Autodesk Inventor part; units mm, degrees
ref_plane "YZ Plane" through (0, 0, 0) normal (1, 0, 0) x (0, 1, 0)
ref_plane "XZ Plane" through (0, 0, 0) normal (0, 1, 0) x (-1, 0, 0)
ref_plane "XY Plane" through (0, 0, 0) normal (0, 0, 1) x (1, 0, 0)
sketch "Sketch1" plane through (0, 0, 0) normal (0, 1, 0) x (-1, 0, 0)
  line L0 (0, 0) -> (-25, 0)
  line L1 (-25, 0) -> (-25, 25)
  line L2 (-25, 25) -> (0, 25)
  line L3 (0, 25) -> (0, 0)
  circle A0 centre (-4.5, 4.5) radius 3
  circle A1 centre (-4.5, 20.5) radius 3
  circle A2 centre (-20.5, 20.5) radius 3
  circle A3 centre (-20.5, 4.5) radius 3
  dimension "d0" = 25
  dimension "d1" = 25
  dimension "d8" = 6
  dimension "d9" = 6
  dimension "d10" = 6
  dimension "d11" = 6
extrude "Extrusion1" add sketch "Sketch1" along normal blind 1 contours L0 L1 L2 L3 | A0 | A1 | A2 | A3
sketch "Sketch2" plane through (0, 1, 0) normal (0, 1, 0) x (1, 0, 0)
  line L0 (10, -12.5) -> (10, -15)
  line L1 (10, -15) -> (12.5, -15)
  line L2 (10, -12.5) -> (10, -10)
  line L3 (10, -10) -> (12.5, -10)
  line L4 (15, -12.5) -> (15, -15)
  line L5 (15, -15) -> (12.5, -15)
  line L6 (15, -12.5) -> (15, -10)
  line L7 (15, -10) -> (12.5, -10)
  point P0 (0, 0)
  dimension "d18" = 2.5
  dimension "d19" = 2.5
  dimension "d20" = 2.5
  dimension "d21" = 2.5
  dimension "d22" = 2.5
  dimension "d23" = 2.5
extrude "Extrusion2" add sketch "Sketch2" along normal blind 0.5
sketch "Sketch6" plane through (0, 1, 0) normal (0, 1, 0) x (1, 0, 0)
  circle A0 centre (4.5, -4.5) radius 4
  circle A1 centre (20.5, -4.5) radius 4
  circle A2 centre (4.5, -20.5) radius 4
  circle A3 centre (20.5, -20.5) radius 4
  point P0 (0, 0)
  dimension "d43" = 8
  dimension "d44" = 8
  dimension "d45" = 8
  dimension "d46" = 8
extrude "Extrusion4" add sketch "Sketch6" along normal blind 0.25
sketch "Sketch7" plane through (4.5, 1.25, 20.5) normal (0, 1, 0) x (1, 0, 0)
  circle A0 centre (0, 0) radius 3
  point P0 (-4.5, 20.5)
  dimension "d49" = 6
hole "Hole2" at (4.5, 1.25, 20.5) direction (0, -1, 0) diameter 6 depth 1.25
sketch "Sketch8" plane through (4.5, 1.25, 4.5) normal (0, 1, 0) x (1, 0, 0)
  circle A0 centre (0, 0) radius 3
  point P0 (-4.5, 4.5)
  dimension "d57" = 6
hole "Hole3" at (4.5, 1.25, 4.5) direction (0, -1, 0) diameter 6 depth 1.25
sketch "Sketch9" plane through (20.5, 1.25, 20.5) normal (0, 1, 0) x (1, 0, 0)
  circle A0 centre (0, 0) radius 3
  point P0 (-20.5, 20.5)
  dimension "d65" = 6
hole "Hole4" at (20.5, 1.25, 20.5) direction (0, -1, 0) diameter 6 depth 1.25
sketch "Sketch10" plane through (20.5, 1.25, 4.5) normal (0, 1, 0) x (1, 0, 0)
  circle A0 centre (0, 0) radius 3
  point P0 (-20.5, 4.5)
  dimension "d73" = 6
hole "Hole5" at (20.5, 1.25, 4.5) direction (0, -1, 0) diameter 6 depth 1.25
properties part number "SiPM"
Can you work these out from the model? Positions are in its coordinate system, mm. A direction names the side the tool comes from. Coordinates: 2 decimals unless noted, no trailing zeros. Loops run counter-clockwise (first coordinate to the right, second up) from the corner with the lowest first, then second, coordinate; pieces in that order, holes last. Notation, with made-up numbers: (31.25, 1.5) -> (62.25, 1.5) arc R5 ccw to (62.25, 9.5) -> close; hole circle Ø2 at (-10, -21). An arc over 180 degrees is marked (long way). Put each result on its own line as item: value. Start each with the question number.
Q1. I'm going to push flat-ended pins straight in: P1, Ø1, axis at x = 10, z = 5.5, coming from the -Y side; P2, Ø4, axis at x = 6, z = 19.5, coming from the +Y side; P3, Ø2.5, axis at x = 19.5, z = 20.5, coming from the +Y side (1 decimal); P4, Ø1, axis at x = 4, z = 9.5, coming from the +Y side. Where does each tip first touch, or does it pass through?
Q2. I want a section at A-A (z = 4.5). Write out the boundary of the cut face in (x, y), plus the area to 3 significant figures.
Q3. If I drill on line 1 (Z direction, x = 4.5, y = 0.9); line 2 (X direction, y = 0.45, z = 2), over which ranges is the centre line in solid material (lowest first)? Write a range as [from, to].
Q4. I want a section at D-D (z = 12). Write out the boundary of the cut face in (x, y), plus the area to 3 significant figures.
Q5. I want a section at C-C (y = 0.35). Write out the boundary of the cut face in (x, z), plus the area to 3 significant figures.
Q6. I want a section at B-B (x = 4.5). Write out the boundary of the cut face in (y, z).
Q7. For faces 1 (the face through (15.5, 1, 12.7)), 2 (the face through (25, 0.5, 12.3)), which set-ups out of +Z, -Z, +X, -X, +Y, -Y let a thin tool reach every point of the face, with its end or its side?
Q8. Thinking about a two-plate mould opening in X: for faces 3 (the face through (12.3, 0.5, 0)), 4 (the face through (0, 0.5, 12.7)), 5 (the face through (22.3, 0.6, 18.1)), which applies, pulls with the +X half, pulls with the -X half, needs draft (parallel to the pull), parting line crosses it, or undercut?
Taken from the geometry:
1. P1: stops at y = 0
1. P2: stops at y = 1.25
1. P3: passes through
1. P4: stops at y = 1
2. outline: (0, 0) -> (1.5, 0) -> (1.5, 1.25) -> (0.5, 1.25) -> (0.5, 1) -> (0, 1) -> close; (7.5, 0) -> (17.5, 0) -> (17.5, 1.25) -> (16.5, 1.25) -> (16.5, 1) -> (8.5, 1) -> (8.5, 1.25) -> (7.5, 1.25) -> close; (23.5, 0) -> (25, 0) -> (25, 1) -> (24.5, 1) -> (24.5, 1.25) -> (23.5, 1.25) -> close
2. area: 14.0 mm2
3. line 1: z = [0, 1.5], [7.5, 17.5], [23.5, 25]
3. line 2: x = [0, 2.84], [6.16, 18.84], [22.16, 25]
4. outline: (0, 0) -> (25, 0) -> (25, 1) -> (15, 1) -> (15, 1.5) -> (10, 1.5) -> (10, 1) -> (0, 1) -> close
4. area: 27.5 mm2
5. outline: (0, 0) -> (25, 0) -> (25, 25) -> (0, 25) -> close; hole circle Ø6 at (4.5, 4.5); hole circle Ø6 at (4.5, 20.5); hole circle Ø6 at (20.5, 4.5); hole circle Ø6 at (20.5, 20.5)
5. area: 512 mm2
6. outline: (0, 0) -> (1, 0) -> (1, 0.5) -> (1.25, 0.5) -> (1.25, 1.5) -> (0, 1.5) -> close; (0, 7.5) -> (1.25, 7.5) -> (1.25, 8.5) -> (1, 8.5) -> (1, 16.5) -> (1.25, 16.5) -> (1.25, 17.5) -> (0, 17.5) -> close; (0, 23.5) -> (1.25, 23.5) -> (1.25, 24.5) -> (1, 24.5) -> (1, 25) -> (0, 25) -> close
7. face 1: +Y
7. face 2: +Z, -Z, +X, +Y, -Y
8. face 3: needs draft
8. face 4: pulls with the -X half
8. face 5: undercut
